```python
from build123d import *

# Parameters (mm, degrees)
EXTRUDE_1_DEPTH     = 16
F_1_0MM_1_D         = 2.6
F_1_0MM_2_D         = 2.6
SKETCH_8_W          = 86.7
SKETCH_8_H          = 16
EXTRUDE_2_DEPTH     = 21.2
SKETCH_9_W          = 86.7
SKETCH_9_H          = 10.4
EXTRUDE_3_DEPTH     = 9.7
SKETCH_15_W         = 20.6
SKETCH_15_H         = 2
EXTRUDE_8_DEPTH     = 13.5
SKETCH_16_W         = 20.6
SKETCH_16_H         = 2
EXTRUDE_9_DEPTH     = 10.5
SKETCH_19_W         = 51.4
SKETCH_19_H         = 10.4
EXTRUDE_10_DEPTH    = 50
SKETCH_25_W         = 50
SKETCH_25_H         = 10.4
EXTRUDE_11_DEPTH    = 45
EXTRUDE_12_DEPTH    = 32
CUT_EXTRUDE_1_DEPTH = 5
SKETCH_29_W         = 51.4
SKETCH_29_H         = 10.402970243
EXTRUDE_13_DEPTH    = 40
SKETCH_32_W         = 40
SKETCH_32_H         = 10.402970243
EXTRUDE_14_DEPTH    = 10
SKETCH_33_W         = 40
SKETCH_33_H         = 10.402970243
EXTRUDE_15_DEPTH    = 10
SKETCH_34_R         = 3
EXTRUDE_16_DEPTH    = 18
F_1_0MM_3_D         = 2.6
F_1_0MM_4_D         = 2.6
FILLET_1_R          = 10
FILLET_2_R          = 10
SKETCH_40_W         = 6
SKETCH_40_H         = 4
EXTRUDE_17_DEPTH    = 11.5
SKETCH_42_W         = 6
SKETCH_42_H         = 19.4
EXTRUDE_18_DEPTH    = 2
SKETCH_46_W         = 60.1
SKETCH_46_H         = 4
EXTRUDE_19_DEPTH    = 2


with BuildPart() as part:
    # 草图1 → 凸台-拉伸1 (new body)
    with BuildSketch(Plane.XY):
        Polygon((-21.523113208, 25.59839861), (-42.123113208, 25.59839861), (-42.123113208, 5.59839861), (44.576886792, 5.59839861), (44.576886792, 25.59839861), (23.976886792, 25.59839861), (23.976886792, 13.12839861), (-21.523113208, 13.12839861), align=None)
    extrude_1 = extrude(amount=EXTRUDE_1_DEPTH)

    # Ø1.0mm 暗销孔1 (through all)
    with Locations(Plane(origin=(0, 25.59839861, 0), x_dir=(1, 0, 0), z_dir=(0, 1, 0))):
        with Locations((36.576886792, -8)):
            f_1_0mm_1 = Hole(F_1_0MM_1_D / 2)

    # Ø1.0mm 暗销孔2 (through all)
    with Locations(Plane(origin=(0, 25.59839861, 0), x_dir=(1, 0, 0), z_dir=(0, 1, 0))):
        with Locations((-34.123113208, -8)):
            f_1_0mm_2 = Hole(F_1_0MM_2_D / 2)

    # 草图8 → 凸台-拉伸2 (add)
    with BuildSketch(Plane.XZ.offset(-5.59839861)):
        with Locations((1.226886792, 8)):
            Rectangle(SKETCH_8_W, SKETCH_8_H)
    extrude_2 = extrude(amount=EXTRUDE_2_DEPTH)

    # 草图9 → 凸台-拉伸3 (add)
    with BuildSketch(Plane(origin=(0, 0, 0), x_dir=(-1, 0, 0), z_dir=(0, 0, -1))):
        with Locations((-1.226886792, -10.40160139)):
            Rectangle(SKETCH_9_W, SKETCH_9_H)
    extrude_3 = extrude(amount=EXTRUDE_3_DEPTH)

    # 草图15 → 凸台-拉伸8 (add)
    with BuildSketch(Plane(origin=(0, -5.20160139, 0), x_dir=(1, 0, 0), z_dir=(0, 1, 0))):
        with Locations((-31.823113208, 8.7)):
            Rectangle(SKETCH_15_W, SKETCH_15_H)
    extrude_8 = extrude(amount=EXTRUDE_8_DEPTH)

    # 草图16 → 凸台-拉伸9 (add)
    with BuildSketch(Plane(origin=(0, 0, -9.7), x_dir=(-1, 0, 0), z_dir=(0, 0, -1))):
        with Locations((31.823113208, 7.29839861)):
            Rectangle(SKETCH_16_W, SKETCH_16_H)
    extrude_9 = extrude(amount=-EXTRUDE_9_DEPTH)

    # 镜向20: 凸台-拉伸1, Ø1.0mm 暗销孔1, Ø1.0mm 暗销孔2, 凸台-拉伸2, 凸台-拉伸3, 凸台-拉伸8, 凸台-拉伸9 across plane
    add(extrude_1.mirror(Plane.XY.offset(-9.7)))
    add(f_1_0mm_1.mirror(Plane.XY.offset(-9.7)), mode=Mode.SUBTRACT)
    add(f_1_0mm_2.mirror(Plane.XY.offset(-9.7)), mode=Mode.SUBTRACT)
    add(extrude_2.mirror(Plane.XY.offset(-9.7)))
    add(extrude_3.mirror(Plane.XY.offset(-9.7)))
    add(extrude_8.mirror(Plane.XY.offset(-9.7)))
    add(extrude_9.mirror(Plane.XY.offset(-9.7)))

    # 草图19 → 凸台-拉伸10 (add)
    with BuildSketch(Plane(origin=(44.576886792, 0, 0), x_dir=(0, 0, -1), z_dir=(1, 0, 0))):
        with Locations((9.7, -10.40160139)):
            Rectangle(SKETCH_19_W, SKETCH_19_H)
    extrude(amount=EXTRUDE_10_DEPTH)

    # 草图25 → 凸台-拉伸11 (add)
    with BuildSketch(Plane(origin=(0, 0, -35.4), x_dir=(-1, 0, 0), z_dir=(0, 0, -1))):
        with Locations((-69.576886792, -10.40160139)):
            Rectangle(SKETCH_25_W, SKETCH_25_H)
    extrude(amount=EXTRUDE_11_DEPTH)

    # 草图26 → 凸台-拉伸12 (add)
    with BuildSketch(Plane(origin=(0, -5.20160139, 0), x_dir=(1, 0, 0), z_dir=(0, 1, 0))):
        Polygon((83.176886792, -9), (94.576886792, -9), (94.576886792, -5), (94.576886792, 80.4), (90.576886792, 80.4), (90.576886792, -5), (83.176886792, -5), align=None)
        Polygon((83.176886792, 28), (84.576886792, 28), (84.576886792, 68), (83.176886792, 68), (81.776886792, 68), (81.776886792, 28), align=None)
    extrude(amount=EXTRUDE_12_DEPTH)

    # 草图28 → 切除-拉伸1 (cut)
    with BuildSketch(Plane(origin=(0, -5.20160139, 0), x_dir=(1, 0, 0), z_dir=(0, 1, 0))):
        Polygon((90.576886792, -5), (84.576886792, -5), (82.576886792, -5), (82.576886792, 28), (84.576886792, 28), (84.576886792, 80.4), (90.576886792, 80.4), align=None)
    extrude(amount=-CUT_EXTRUDE_1_DEPTH, mode=Mode.SUBTRACT)

    # 草图29 → 凸台-拉伸13 (add)
    with BuildSketch(Plane.ZY.offset(42.123113208)):
        with Locations((-9.7, -10.400116268)):
            Rectangle(SKETCH_29_W, SKETCH_29_H)
    extrude(amount=EXTRUDE_13_DEPTH)

    # 草图32 → 凸台-拉伸14 (add)
    with BuildSketch(Plane(origin=(0, 0, -35.4), x_dir=(-1, 0, 0), z_dir=(0, 0, -1))):
        with Locations((62.123113208, -10.400116268)):
            Rectangle(SKETCH_32_W, SKETCH_32_H)
    extrude(amount=EXTRUDE_14_DEPTH)

    # 草图33 → 凸台-拉伸15 (add)
    with BuildSketch(Plane.XY.offset(16)):
        with Locations((-62.123113208, -10.400116268)):
            Rectangle(SKETCH_33_W, SKETCH_33_H)
    extrude(amount=EXTRUDE_15_DEPTH)

    # 草图34 → 凸台-拉伸16 (add)
    with BuildSketch(Plane(origin=(0, -5.198631147, 0), x_dir=(1, 0, 0), z_dir=(0, 1, 0))):
        with Locations(Location((-52.123113208, 38.7, 0), (0, 0, 90))):
            Circle(SKETCH_34_R)
        with Locations(Location((-75.123113208, 38.7, 0), (0, 0, 90))):
            Circle(SKETCH_34_R)
        with Locations(Location((-52.123113208, -19.3, 0), (0, 0, 90))):
            Circle(SKETCH_34_R)
        with Locations(Location((-75.123113208, -19.3, 0), (0, 0, 90))):
            Circle(SKETCH_34_R)
    extrude(amount=EXTRUDE_16_DEPTH)

    # Ø1.0mm 暗销孔3 (through all)
    with Locations(Plane(origin=(0, 12.801368853, 0), x_dir=(1, 0, 0), z_dir=(0, 1, 0))):
        with Locations((-52.123113208, 38.7)):
            Hole(F_1_0MM_3_D / 2)

    # Ø1.0mm 暗销孔4 (through all)
    with Locations(Plane(origin=(0, 12.801368853, 0), x_dir=(1, 0, 0), z_dir=(0, 1, 0))):
        with Locations((-52.123113208, -19.3), (-75.123113208, 38.7), (-75.123113208, -19.3)):
            Hole(F_1_0MM_4_D / 2)

    # 圆角1
    fillet_1_edges = [part.edges().sort_by_distance(p)[0] for p in [
        (44.576886792, -10.40160139, -80.4),
        (94.576886792, -10.40160139, 16),
        (-42.123113208, -10.400116268, -45.4),
        (-42.123113208, -10.400116268, 26),
        (-82.123113208, -10.400116268, -45.4),
        (-82.123113208, -10.400116268, 26),
    ]]
    fillet(fillet_1_edges, radius=FILLET_1_R - 0.0001)  # a hair under: the kernel refuses the full size

    # 圆角2
    fillet_2_edges = [part.edges().sort_by_distance(p)[0] for p in [
        (94.576886792, 5.59839861, -80.4),
    ]]
    fillet(fillet_2_edges, radius=FILLET_2_R - 0.0001)  # a hair under: the kernel refuses the full size

    # 草图40 → 凸台-拉伸17 (add)
    with BuildSketch(Plane(origin=(0, -5.20160139, 0), x_dir=(1, 0, 0), z_dir=(0, 1, 0))):
        with Locations((41.576886792, 9.7)):
            Rectangle(SKETCH_40_W, SKETCH_40_H)
    extrude(amount=EXTRUDE_17_DEPTH)

    # 草图42 → 凸台-拉伸18 (add)
    with BuildSketch(Plane(origin=(0, 6.29839861, 0), x_dir=(1, 0, 0), z_dir=(0, 1, 0))):
        with Locations((41.576886792, 9.7)):
            Rectangle(SKETCH_42_W, SKETCH_42_H)
    extrude(amount=EXTRUDE_18_DEPTH)

    # 草图46 → 凸台-拉伸19 (add)
    with BuildSketch(Plane(origin=(0, -5.20160139, 0), x_dir=(1, 0, 0), z_dir=(0, 1, 0))):
        with Locations((8.526886792, 9.7)):
            Rectangle(SKETCH_46_W, SKETCH_46_H)
    extrude(amount=EXTRUDE_19_DEPTH)


solid = part.part
```
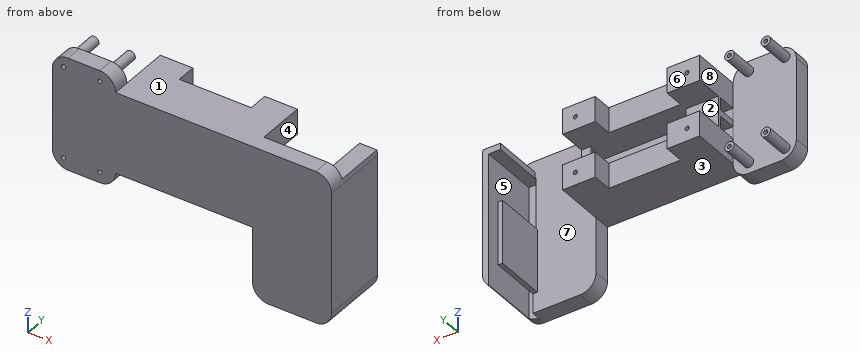
Geometry check sheet. Reference: the model listing, model coordinates, mm. Face numbers are marked on the shaded views. A direction names the side the tool comes from. Round coordinates to 2 decimals unless told otherwise and drop trailing zeros. Loops run counter-clockwise (first coordinate to the right, second up) from the corner with the lowest first, then second, coordinate; pieces in that order, holes last. Notation, with made-up numbers: (27, 58.25) - (72, 58.25) arc R21 ccw to (72, 65.25) - close; hole circle Ø9 at (43.5, 27.5). An arc over 180 degrees is marked (long way). Write item = value, one per line. Start each with the question number.
1. Section check A-A on z = -4. Give the number of separate pieces and of enclosed holes in the cut face, then the cut area to 3 significant figures.
2. Section check D-D on x = 20.5. Enter the section's corners in (y, z).
3. Section check B-B on x = -37.5. Enter the section's corners in (y, z), then the cut area to 3 significant figures.
4. Section check C-C on z = -31.5. Enter the section's corners in (x, y).
5. Mould release check, pull along X, two halves, no side actions. Record for the marked faces 6, 7 and 8: released by +X, released by -X, zero draft, split by the parting line, or undercut.
6. Set-up check for the marked faces 1, 2, 3, 4 and 5: record each of +Z, -Z, +X, -X, +Y, -Y from which the full face is reachable in a straight line by a thin tool's end or side.
7. Depth check by flat-ended pin: pin 1 (1.3 mm diameter, centred on x = -34, z = 8, fed in from +Y); pin 2 (9 mm diameter, centred on y = 3, z = -7, fed in from -X); pin 3 (5 mm diameter, centred on x = -31, z = -30.5, fed in from +Y); pin 4 (2 mm diameter, centred on x = -52.12, z = -38.7, fed in from -Y). Enter the tip coordinate at first touch or a pass-through.
8. Thickness scan on line 1 (X direction, y = -2.25, z = 19.3); line 2 (X direction, y = -1.5, z = -33); line 3 (Z direction, x = -52, y = 5). Record the ranges inside material, lowest first.
Working result:
q1.separate_pieces = 3
q1.enclosed_holes = 0
q1.area = 1,980 mm^2
q2.outline = (-15.6, -35.4) - (13.13, -35.4) - (13.13, -19.4) - (-5.2, -19.4) - (-5.2, -11.7) - (-3.2, -11.7) - (-3.2, -7.7) - (-5.2, -7.7) - (-5.2, 0) - (13.13, 0) - (13.13, 16) - (-15.6, 16) - close
q3.outline = (-15.6, -35.4) - (25.6, -35.4) - (25.6, -19.4) - (8.3, -19.4) - (8.3, 0) - (25.6, 0) - (25.6, 16) - (-15.6, 16) - close; hole (-5.2, -19.4) - (6.3, -19.4) - (6.3, -11.7) - (-5.2, -11.7) - close; hole (-5.2, -7.7) - (6.3, -7.7) - (6.3, 0) - (-5.2, 0) - close
q3.area = 1,600 mm^2
q4.outline = (-82.12, -15.6) - (94.58, -15.6) - (94.58, 26.8) - (90.58, 26.8) - (90.58, -10.2) - (84.58, -10.2) - (84.58, 26.8) - (81.78, 26.8) - (81.78, -5.2) - (44.58, -5.2) - (44.58, 25.6) - (23.98, 25.6) - (23.98, 13.13) - (-21.52, 13.13) - (-21.52, 25.6) - (-42.12, 25.6) - (-42.12, -5.2) - (-82.12, -5.2) - close
q5.face_6 = zero draft
q5.face_7 = undercut
q5.face_8 = released by -X
q6.face_1 = +Z, +X, +Y, -Y
q6.face_2 = -X, +Y
q6.face_3 = -Z, +Y, -Y
q6.face_4 = +Z, -Z, +Y
q6.face_5 = -Z, +Y
q7.pin_1 = 5.6
q7.pin_2 = -42.12
q7.pin_3 = 25.6
q7.pin_4 = through
q8.line_1 = -78.12 to -76.42, -73.82 to -72.12, -55.12 to -53.42, -50.82 to -49.12
q8.line_2 = -42.12 to 44.58, 81.78 to 84.58, 90.58 to 94.58
q8.line_3 = -41.7 to -39.99, -37.41 to -35.7, 16.3 to 18.01, 20.59 to 22.3
